Autodesk Inventor part; units mm, degrees
ref_plane "YZ Plane" through (0, 0, 0) normal (1, 0, 0) x (0, 1, 0)
ref_plane "XZ Plane" through (0, 0, 0) normal (0, 1, 0) x (-1, 0, 0)
ref_plane "XY Plane" through (0, 0, 0) normal (0, 0, 1) x (1, 0, 0)
sketch "스케치1" plane through (0, 0, 0) normal (0, 0, 1) x (1, 0, 0)
  line L0 (-9.8208, 11.7001) -> (11.3566, 11.7001)
  line L1 (11.3566, 11.7001) -> (11.3566, -10.0835)
  line L2 (11.3566, -10.0835) -> (-9.8208, -10.0835)
  line L3 (-9.8208, -10.0835) -> (-9.8208, 11.7001)
  point P0 (0, 0)
extrude "돌출1" add sketch "스케치1" along normal blind 25
sketch "스케치2" plane through (11.3566, -10.0835, 0) normal (1, 0, 0) x (0, 0, -1)
  line L0 (0, 0) -> (-25, 0)
  line L1 (-18.1058, 4.6881) -> (-6.628, 4.6881)
  line L2 (-6.628, 4.6881) -> (-6.628, 0)
  line L3 (-6.628, 0) -> (-18.1058, 0)
  line L4 (-18.1058, 0) -> (-18.1058, 4.6881)
  point P0 (0, 10.0835)
extrude "돌출2" cut sketch "스케치2" against normal blind 25
sketch "스케치3" plane through (11.3566, -10.0835, 0) normal (1, 0, 0) x (0, 0, -1)
  line L0 (0, 21.7836) -> (-25, 21.7836)
  line L1 (-18.1058, 21.7836) -> (-6.6684, 21.7836)
  line L2 (-6.6684, 21.7836) -> (-6.6684, 13.7006)
  line L3 (-6.6684, 13.7006) -> (-18.1058, 13.7006)
  line L4 (-18.1058, 13.7006) -> (-18.1058, 21.7836)
  point P0 (0, 10.0835)
extrude "돌출3" cut sketch "스케치3" against normal blind 25
sketch "스케치4" plane through (11.3566, -10.0835, 0) normal (1, 0, 0) x (0, 0, -1)
  point P0 (0, 10.0835)
sketch "스케치5" plane through (-9.8208, 11.7001, 0) normal (0, 1, 0) x (1, 0, 0)
  line L0 (21.1774, -6.628) -> (0, -6.628)
  line L1 (0, 0) -> (21.1774, 0)
  line L2 (4.1053, -6.628) -> (17.5214, -6.628)
  line L3 (17.5214, -6.628) -> (17.5214, 0)
  line L4 (17.5214, 0) -> (4.1053, 0)
  line L5 (4.1053, 0) -> (4.1053, -6.628)
  point P0 (9.8208, 0)
sketch "스케치6" plane through (11.3566, 3.6171, 6.6684) normal (0, 0, 1) x (1, 0, 0)
  line L0 (-21.1774, 8.083) -> (0, 8.083)
  line L1 (0, 0) -> (-21.1774, 0)
  line L2 (-16.9228, 8.083) -> (-3.828, 8.083)
  line L3 (-3.828, 8.083) -> (-3.828, 0)
  line L4 (-3.828, 0) -> (-16.9228, 0)
  line L5 (-16.9228, 0) -> (-16.9228, 8.083)
  point P0 (-11.3566, -3.6171)
extrude "돌출4" cut sketch "스케치6" against normal blind 10
sketch "스케치7" plane through (11.3566, -10.0835, 0) normal (1, 0, 0) x (0, 0, -1)
  line L0 (-6.6684, 13.7006) -> (-18.1058, 13.7006)
  line L1 (0, 21.7836) -> (0, 13.7006)
  line L2 (-6.6684, 13.7006) -> (0, 21.7836)
  line L3 (-6.6684, 13.7006) -> (-6.6684, 21.7836)
  line L4 (0, 21.7836) -> (0, 0)
  line L5 (-6.6684, 21.7836) -> (0, 21.7836)
  point P0 (0, 10.0835)
extrude "돌출5" cut sketch "스케치7" against normal blind 50
sketch "스케치8" plane through (11.3566, -10.0835, 25) normal (1, 0, 0) x (0, 0, -1)
  line L0 (0, 21.7836) -> (0, 0)
  line L1 (6.8942, 13.7006) -> (18.3316, 13.7006)
  line L2 (0, 21.7836) -> (6.8942, 13.7006)
  line L3 (6.8942, 21.7836) -> (6.8942, 13.7006)
  line L4 (6.8942, 13.7006) -> (6.8942, 21.7836)
  line L5 (6.8942, 21.7836) -> (0, 21.7836)
  line L6 (6.8942, 21.7836) -> (0, 21.7836)
  point P0 (25, 10.0835)
extrude "돌출6" cut sketch "스케치8" against normal blind 15
properties part number "240510_3Dsketch09"
Work out the finished part from the listing and answer in its coordinate system (mm). A direction names the side the tool comes from. Round coordinates to 2 decimals unless told otherwise and drop trailing zeros. Loops run counter-clockwise (first coordinate to the right, second up) from the corner with the lowest first, then second, coordinate; pieces in that order, holes last.
(1) The part is cut by section D-D, the plane x = -4.5. Give the vertices of the cut face in (y, z), and give its area (3 significant figures).
Computed values:
outline: (-10.08, 0) - (3.62, 0) - (3.62, 18.11) - (11.7, 18.11) - (11.7, 25) - (-10.08, 25) - (-10.08, 18.11) - (-5.4, 18.11) - (-5.4, 6.63) - (-10.08, 6.63) - close
area: 344 mm2
(2) The part is cut by section B-B, the plane x = 6. Give the vertices of the cut face in (y, z).
Computed values:
outline: (-10.08, 0) - (3.62, 0) - (3.62, 18.11) - (11.7, 25) - (-10.08, 25) - (-10.08, 18.11) - (-5.4, 18.11) - (-5.4, 6.63) - (-10.08, 6.63) - close
(3) The part is cut by section C-C, the plane z = 3.75. Give the vertices of the cut face in (x, y), and give its area (3 significant figures).
Computed values:
outline: (-9.82, -10.08) - (11.36, -10.08) - (11.36, 7.15) - (7.53, 7.15) - (7.53, 3.62) - (-5.57, 3.62) - (-5.57, 7.15) - (-9.82, 7.15) - close
area: 319 mm2
(4) The part is cut by section A-A, the plane y = 10.75. Give the vertices of the cut face in (x, z), and give its area (3 significant figures).
Computed values:
outline: (-9.82, 0) - (-5.57, 0) - (-5.57, 0.78) - (-9.82, 0.78) - close; (-9.82, 18.11) - (-3.64, 18.11) - (-3.64, 24.19) - (11.36, 24.19) - (11.36, 25) - (-9.82, 25) - close; (7.53, 0) - (11.36, 0) - (11.36, 0.78) - (7.53, 0.78) - close
area: 61.1 mm2
(5) Find the intervals of material crossed by L1, parallel to Z at x = -0.5, y = -7.5; L2, parallel to Y at x = 3, z = 7.25; L3, parallel to Z at x = -5.25, y = 9.5, in increasing order.
Computed values:
L1: z = 0 to 6.63, 18.11 to 25
L2: y = -5.4 to 3.62
L3: z = 18.11 to 25
(6) For faces 1 (the flat face through (7.529, 6, 2)), 2 (the flat face through (-7, 8, 18.106)), 3 (the flat face through (3.962, 7.715, 21.601)), 4 (the flat face through (1, -8, 18.106)), determine the directions among +Z, -Z, +X, -X, +Y, -Y from which every point of the face is accessible in a straight line to the end or side of a thin tool.
Computed values:
face 1: -Z, +Y
face 2: +X, -X, +Y
face 3: +X, +Y
face 4: +X, -X, -Y
(7) This flat-tipped pin is pushed along its axis until it touches: P1, Ø8, axis at x = 8.5, z = 13, coming from the -Y side. Where does it stop, or does it pass through?
Computed values:
P1: stops at y = -5.4
(8) The mould has two halves that part along X. Classify faces 5 (the flat face through (1, -1, 0)), 6 (the flat face through (-9.821, 1, 12)), 7 (the flat face through (-5.566, 6, 2)): pulls with the +X half, pulls with the -X half, needs draft (parallel to the pull), parting line crosses it, or undercut.
Computed values:
face 5: needs draft
face 6: pulls with the -X half
face 7: undercut
